```python
from build123d import *

# Parameters (mm, degrees)
SKETCH1_R           = 1.5
BOSS_EXTRUDE1_DEPTH = 3
SKETCH2_R           = 1.5
SKETCH2_W           = 86
SKETCH2_H           = 51
BOSS_EXTRUDE2_DEPTH = 4
BOSS_EXTRUDE3_DEPTH = 20
SKETCH4_W           = 4
SKETCH4_H           = 56
BOSS_EXTRUDE4_DEPTH = 8
SKETCH5_R           = 1.45
CUT_EXTRUDE1_DEPTH  = 120.837389825


with BuildPart() as part:
    # Sketch1 → Boss-Extrude1 (new body)
    with BuildSketch(Plane(origin=(0, 0, 0), x_dir=(1, 0, 0), z_dir=(0, 1, 0))):
        Polygon((0, 0), (94, 0), (100, 0), (100, 6), (94, 6), (94, 50), (100, 50), (100, 56), (94, 56), (0, 56), (-6, 56), (-6, 50), (0, 50), (0, 6), (-6, 6), (-6, 0), align=None)
        with Locations(Location((-3, 53, 0), (0, 0, 270))):
            Circle(SKETCH1_R, mode=Mode.SUBTRACT)
        with Locations(Location((97, 53, 0), (0, 0, 90))):
            Circle(SKETCH1_R, mode=Mode.SUBTRACT)
        with Locations(Location((97, 3, 0), (0, 0, 270))):
            Circle(SKETCH1_R, mode=Mode.SUBTRACT)
        with Locations(Location((-3, 3, 0), (0, 0, 90))):
            Circle(SKETCH1_R, mode=Mode.SUBTRACT)
    extrude(amount=BOSS_EXTRUDE1_DEPTH)

    # Sketch2 → Boss-Extrude2 (add)
    with BuildSketch(Plane(origin=(0, 3, 0), x_dir=(1, 0, 0), z_dir=(0, 1, 0))):
        Polygon((0, 50), (0, 6), (-6, 6), (-6, 0), (100, 0), (100, 6), (94, 6), (94, 50), (100, 50), (100, 56), (-6, 56), (-6, 50), align=None)
        with Locations(Location((-3, 53, 0), (0, 0, 270))):
            Circle(SKETCH2_R, mode=Mode.SUBTRACT)
        with Locations(Location((97, 53, 0), (0, 0, 90))):
            Circle(SKETCH2_R, mode=Mode.SUBTRACT)
        with Locations(Location((97, 3, 0), (0, 0, 270))):
            Circle(SKETCH2_R, mode=Mode.SUBTRACT)
        with Locations(Location((-3, 3, 0), (0, 0, 90))):
            Circle(SKETCH2_R, mode=Mode.SUBTRACT)
        with Locations((47, 28)):
            Rectangle(SKETCH2_W, SKETCH2_H, mode=Mode.SUBTRACT)
    extrude(amount=BOSS_EXTRUDE2_DEPTH)

    # Sketch3 → Boss-Extrude3 (add)
    with BuildSketch(Plane(origin=(0, 7, 0), x_dir=(1, 0, 0), z_dir=(0, 1, 0))):
        Polygon((8, 56), (0, 56), (0, 48), (4, 48), (4, 53.5), (8, 53.5), align=None)
        Polygon((90, 48), (94, 48), (94, 56), (86, 56), (86, 53.5), (90, 53.5), align=None)
        Polygon((94, 0), (94, 8), (90, 8), (90, 2.5), (86, 2.5), (86, 0), align=None)
        Polygon((4, 8), (0, 8), (0, 0), (8, 0), (8, 2.5), (4, 2.5), align=None)
    extrude(amount=BOSS_EXTRUDE3_DEPTH)

    # Sketch4 → Boss-Extrude4 (add)
    with BuildSketch(Plane(origin=(0, 27, 0), x_dir=(1, 0, 0), z_dir=(0, 1, 0))):
        with Locations((2, 28)):
            Rectangle(SKETCH4_W, SKETCH4_H)
        with Locations((92, 28)):
            Rectangle(SKETCH4_W, SKETCH4_H)
    extrude(amount=BOSS_EXTRUDE4_DEPTH)

    # Sketch5 → Cut-Extrude1 (cut, through all)
    with BuildSketch(Plane.ZY):
        with Locations((-52, 31)):
            Circle(SKETCH5_R)
        with Locations((-40, 31)):
            Circle(SKETCH5_R)
        with Locations((-28, 31)):
            Circle(SKETCH5_R)
        with Locations((-16, 31)):
            Circle(SKETCH5_R)
        with Locations((-4, 31)):
            Circle(SKETCH5_R)
    extrude(amount=-CUT_EXTRUDE1_DEPTH, mode=Mode.SUBTRACT)


solid = part.part
```
Geometry: final body of the model. Coordinates: model frame, mm. A direction names the side the tool comes from. Round coordinates to 2 decimals unless told otherwise and drop trailing zeros. Order: outer loops, then holes, each group sorted by start corner. A loop starts at its lowest first (then second) coordinate and runs counter-clockwise, first axis right, second up. Notation, with made-up numbers: (-3, -26.5) - (46, -26.5) arc R24 cw to (46, -9.5) - close; hole circle Ø4 at (86.5, 12.5). An arc over 180 degrees is marked (long way). Use CSV: the item, a comma, the result in double quotes. Start each with the question number.
Q1. Section query B-B (z = -25.5). Return loops of the section in (x, y), and give its area (3 significant figures).
Q2. Section query C-C (z = -16). Return loops of the section in (x, y), and give its area (3 significant figures).
Q3. Access query for faces 1 (the face through (88, 27, -1)), 2 (the face through (-3, 3, -50)), 3 (the face through (4, 29, -28)). Directions: +Z, -Z, +X, -X, +Y, -Y. A direction counts if a zero-diameter tool reaches every point of the face in a straight line with its end or side. Return the directions, or none.
Q4. Section query A-A (y = 20.5). Return loops of the section in (x, z), and give its area (3 significant figures).
Q5. Mould query, pull axis Y, two halves, no side actions, for faces 4 (the face through (1.97, 30.12, -53.15)), 5 (the face through (-4.4, 7, -4.4)), 6 (the face through (98.487, 3.451, -3.195)). Classes: +Y half, -Y half, draft (parallel to the pull), parting line (faces both ways), or undercut.
Q6. Material intervals for line 1 along Y through (x, z) = (3, -28); line 2 along X through (y, z) = (33.5, -9); line 3 along Z through (x, y) = (3, 16), sorted ascending. Write a range as from..to.
Q7. Section query D-D (x = 73.5). Return loops of the section in (y, z).
Q8. First-contact query: pin 1 (3 mm diameter, centred on y = 31, z = -19.5, fed in from -X); pin 2 (1.5 mm diameter, centred on x = 22, z = -25, fed in from +Y); pin 3 (6 mm diameter, centred on x = 59, y = 9, fed in from +Z); pin 4 (0.8 mm diameter, centred on x = 87, z = -54.5, fed in from +Y). Flat tips, straight axial feed; report the tip coordinate or a pass-through.
Result set:
1,outline,"(0, 0) - (94, 0) - (94, 7) - (90, 7) - (90, 3) - (4, 3) - (4, 7) - (0, 7) - close; (0, 27) - (4, 27) - (4, 35) - (0, 35) - close; (90, 27) - (94, 27) - (94, 35) - (90, 35) - close"
1,area,"378 mm2"
2,outline,"(0, 0) - (94, 0) - (94, 7) - (90, 7) - (90, 3) - (4, 3) - (4, 7) - (0, 7) - close; (0, 27) - (4, 27) - (4, 29.55) - (0, 29.55) - close; (0, 32.45) - (4, 32.45) - (4, 35) - (0, 35) - close; (90, 27) - (94, 27) - (94, 29.55) - (90, 29.55) - close; (90, 32.45) - (94, 32.45) - (94, 35) - (90, 35) - close"
2,area,"355 mm2"
3,face 1,"+Z, -Z, +Y"
3,face 2,"-X, +Y, -Y"
3,face 3,"+Y"
4,outline,"(0, -56) - (8, -56) - (8, -53.5) - (4, -53.5) - (4, -48) - (0, -48) - close; (0, -8) - (4, -8) - (4, -2.5) - (8, -2.5) - (8, 0) - (0, 0) - close; (86, -56) - (94, -56) - (94, -48) - (90, -48) - (90, -53.5) - (86, -53.5) - close; (86, -2.5) - (90, -2.5) - (90, -8) - (94, -8) - (94, 0) - (86, 0) - close"
4,area,"168 mm2"
5,face 4,"undercut"
5,face 5,"+Y half"
5,face 6,"draft"
6,line 1,"y = 0..7, 27..29.55, 32.45..35"
6,line 2,"x = 0..4, 90..94"
6,line 3,"z = -56..-48, -8..0"
7,outline,"(0, -56) - (7, -56) - (7, -53.5) - (3, -53.5) - (3, -2.5) - (7, -2.5) - (7, 0) - (0, 0) - close"
8,pin 1,"stops at x = 0"
8,pin 2,"stops at y = 3"
8,pin 3,"stops at z = 0"
8,pin 4,"stops at y = 27"
